The drawing under review shows one solid part. Ordinate dimensions are in mm from its lowest x, y, z. A direction names the side the tool comes from. Coordinates: 2 decimals unless noted, no trailing zeros. Loops run counter-clockwise (first coordinate to the right, second up) from the corner with the lowest first, then second, coordinate; pieces in that order, holes last. Notation, with made-up numbers: (52, 46) -> (108, 46) arc R3 cw to (108, 50) -> close; hole circle Ø4 at (-25.75, -28). An arc over 180 degrees is marked (long way). Use a Markdown table: item, result.
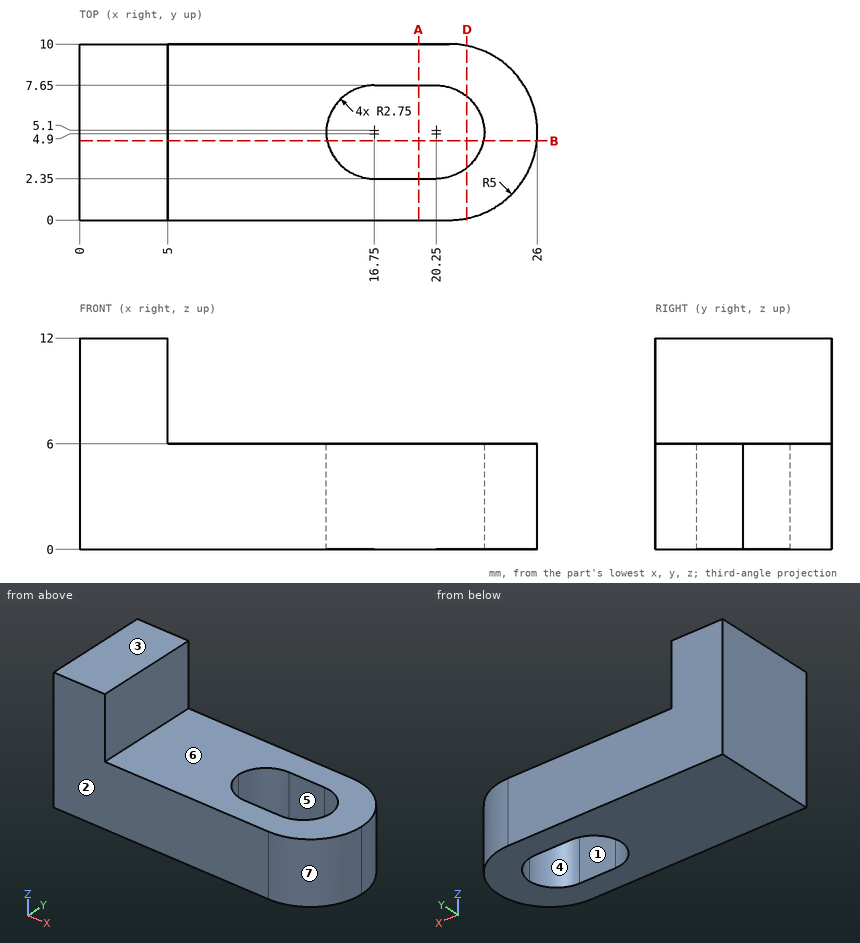
(1) For pin 1 Ø1.8 at (y, z) = (5.5, 8.5) entering from +X; pin 2 Ø1.5 at (x, y) = (7, 4) entering from +Z; pin 3 Ø1 at (y, z) = (7, 3.5) entering from +X, all flat-tipped, find the tip position at first contact; note any pin that passes through.
Found:
| item | result |
|---|---|
| pin 1 | stops at x = 5 |
| pin 2 | stops at z = 6 |
| pin 3 | stops at x = 25.77 |
(2) For line 1 along Z through (x, y) = (11, 1.5); line 2 along Y through (x, z) = (16, 4.25); line 3 along Y through (x, z) = (14.5, 4.75), list the stretches that pass through material, from the lowest coordinate up.
Found:
| item | result |
|---|---|
| line 1 | z = 0 to 6 |
| line 2 | y = 0 to 2.45, 7.55 to 10 |
| line 3 | y = 0 to 3.52, 6.48 to 10 |
(3) Take a section at A-A on x = 19.25. Write out the cut boundary in (y, z), plus the area to 3 significant figures.
Found:
| item | result |
|---|---|
| outline | (0, 0) -> (2.35, 0) -> (2.35, 6) -> (0, 6) -> close; (7.65, 0) -> (10, 0) -> (10, 6) -> (7.65, 6) -> close |
| area | 28.2 mm^2 |
(4) For the marked faces 5, 6 and 7, list the 3-axis set-ups (+Z, -Z, +X, -X, +Y, -Y) from which the entire face can be reached by the end or side of a thin tool; tool diameter is ignored.
Found:
| item | result |
|---|---|
| face 5 | +Z, -Z |
| face 6 | +Z, +X, +Y, -Y |
| face 7 | +Z, -Z, +X, -Y |
(5) Mouldability with a two-part tool opening along Y and no side actions: class the marked faces 1, 2, 3 and 4 as pulls with the +Y half, pulls with the -Y half, needs draft (parallel to the pull), parting line crosses it, or undercut.
Found:
| item | result |
|---|---|
| face 1 | undercut |
| face 2 | pulls with the -Y half |
| face 3 | needs draft |
| face 4 | undercut |
(6) Take a section at D-D on x = 22. Write out the cut boundary in (y, z).
Found:
| item | result |
|---|---|
| outline | (0.1, 0) -> (2.98, 0) -> (2.98, 6) -> (0.1, 6) -> close; (7.02, 0) -> (9.9, 0) -> (9.9, 6) -> (7.02, 6) -> close |
(7) Take a section at B-B on y = 4.5. Write out the cut boundary in (x, z).
Found:
| item | result |
|---|---|
| outline | (0, 0) -> (14.07, 0) -> (14.07, 6) -> (5, 6) -> (5, 12) -> (0, 12) -> close; (22.93, 0) -> (25.97, 0) -> (25.97, 6) -> (22.93, 6) -> close |
